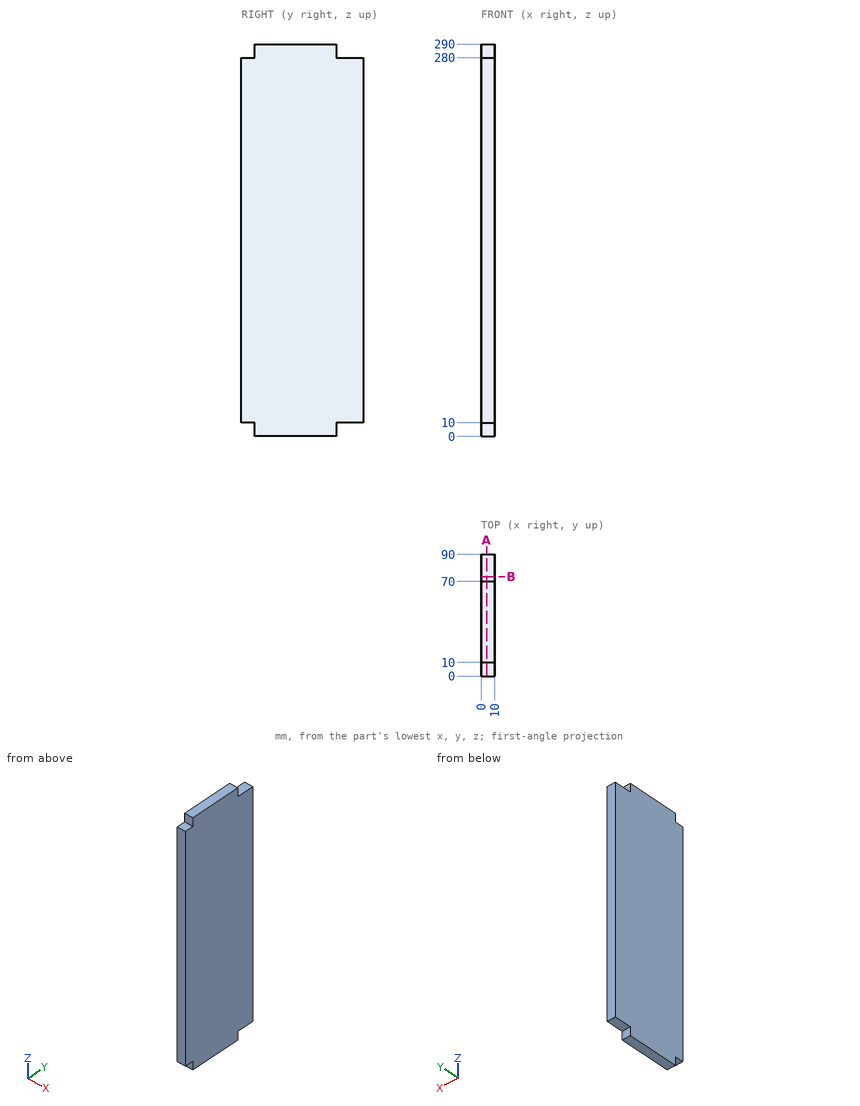
Job drawing, mm, ordinate dimensions from the low corner. One solid piece. Round coordinates to 2 decimals unless told otherwise and drop trailing zeros. Order: outer loops, then holes, each group sorted by start corner. A loop starts at its lowest first (then second) coordinate and runs counter-clockwise, first axis right, second up. Notation, with made-up numbers: M 32.5,31 L 50.5,31 A29 ccw 50.5,66 Z; hole C 29.5,89 d1. An arc over 180 degrees is marked long. Write each question's results on one line, items separated by ' | '. Start each with the question number.
(1) Drop flat-ended pins along their axis: pin 1 (5 mm diameter, centred on x = 7, y = 7, fed in from +Z); pin 2 (5 mm diameter, centred on x = 3.5, z = 284, fed in from -Y). Give the stop position or say it passes through.
(2) Saw through at A-A, the plane x = 4. Give the cut face in (y, z), then the cut area to 3 significant figures.
(3) Saw through at B-B, the plane y = 73.5. Give the cut face in (x, z).
(4) Probe probe 1 along Z at (x, y) = (9.75, 86). List the from-to ranges inside material, lowest first. Write a range as from..to.
Established:
1) pin 1: stops at z = 280 | pin 2: stops at y = 10
2) outline: M 0,10 L 10,10 L 10,0 L 70,0 L 70,10 L 90,10 L 90,280 L 70,280 L 70,290 L 10,290 L 10,280 L 0,280 Z | area: 25,500 mm^2
3) outline: M 0,10 L 10,10 L 10,280 L 0,280 Z
4) probe 1: z = 10..280
